```python
from build123d import *

# Parameters (mm, degrees)
F1_DEPTH    = 15
F2_T1_DEPTH = 34.8219363514
F2_T3_DEPTH = 25.2867319519
F2_T5_DEPTH = 87.7867319519
F3_R        = 5
F4_SIZE     = 1


# Not quite as in the source:
# - a fillet or chamfer that OpenCascade refuses, or shapes differently, is made with other operations: its cross-section is extruded or revolved along the edge and cut away or added


with BuildPart() as f1:
    # F0 (on Front) → F1 (new body)
    with BuildSketch(Plane.XZ):
        with BuildLine():
            Line((50, 60), (0, 60))
            Line((0, 60), (-27.5, 60))
            Line((-27.5, 60), (-27.5, 29.0612040202))
            Line((-27.5, 29.0612040202), (-10.1093475479, 5.1480552127))
            ThreePointArc((-10.1093475479, 5.1480552127), (0, 0), (10.1093475479, 5.1480552127))
            Line((10.1093475479, 5.1480552127), (50, 60))
        make_face()
        with BuildLine():
            ThreePointArc((12.5, 32.5), (-8.8388347648, 23.6611652352), (0, 45))
            ThreePointArc((0, 45), (8.8388347648, 41.3388347648), (12.5, 32.5))
        make_face(mode=Mode.SUBTRACT)
    extrude(amount=F1_DEPTH)

    # F2: chamfer of 2 on 7 edges, made by hand

    # F2_s2 → F2_t1 (cut)
    with BuildSketch(Plane.XZ.offset(-9.9109681757)):
        Polygon((47.69005228, 56.823688834), (46.0725566723, 60), (50, 60), align=None)
    extrude(amount=F2_T1_DEPTH, mode=Mode.SUBTRACT)

    # F2_s4 → F2_t3 (cut)
    with BuildSketch(Plane.XZ.offset(-5.1433659759)):
        Polygon((-25.5, 60), (-27.5, 58), (-27.5, 60), align=None)
    extrude(amount=F2_T3_DEPTH, mode=Mode.SUBTRACT)

    # F2_s6 → F2_t5 (cut)
    with BuildSketch(Plane.YZ.offset(-32.6433659759)):
        Polygon((-2, 60), (0, 58), (0, 60), align=None)
        Polygon((-13, 60), (-15, 58), (-15, 60), align=None)
    extrude(amount=F2_T5_DEPTH, mode=Mode.SUBTRACT)

    # F2_s7 → F2_t8 (revolve, cut)
    with BuildSketch(Plane.XY.offset(32.5)):
        Polygon((12.5, -2), (14.5, 0), (12.5, 0), align=None)
    revolve(axis=Axis((0, 0, 32.5), (0, 1, 0)), mode=Mode.SUBTRACT)

    # F2_s9 → F2_t10 (revolve, cut)
    with BuildSketch(Plane.XY.offset(32.5)):
        Polygon((12.5, -13), (14.5, -15), (12.5, -15), align=None)
    revolve(axis=Axis((0, -15, 32.5), (0, 1, 0)), mode=Mode.SUBTRACT)

    # F3
    f3_edges = [f1.edges().sort_by_distance(p)[0] for p in [
        (-27.5, -7.5, 29.061204),
    ]]
    fillet(f3_edges, radius=F3_R)

    # F4
    f4_edges = [f1.edges().sort_by_distance(p)[0] for p in [
        (28.8997, -15, 30.985872),
        (28.8997, 0, 30.985872),
        (-27.5, 0, 44.343534),
        (-27.254929, 0, 29.140895),
        (-18.326543, 0, 16.447173),
        (0, 0, 0),
        (-27.5, -15, 44.343534),
        (-27.254929, -15, 29.140895),
        (-18.326543, -15, 16.447173),
        (0, -15, 0),
    ]]
    chamfer(f4_edges, length=F4_SIZE)


solid = f1.part
```
For this review, take the finished solid that the model builds, in its own axes (mm). Round coordinates to 2 decimals unless told otherwise and drop trailing zeros. Order: outer loops, then holes, each group sorted by start corner. A loop starts at its lowest first (then second) coordinate and runs counter-clockwise, first axis right, second up.
Q1. Mouldability with a two-part tool opening along Z and no side actions: class faces 1 (the flat face through (46.893, -7.395, 58.39)), 2 (the conical face through (-2.737, -1.875, 44.825)), 3 (the cylindrical face through (-27.26, -7.59, 29.16)), 4 (the conical face through (-2.737, -13.125, 44.825)) as pulls with the +Z half, pulls with the -Z half, needs draft (parallel to the pull), parting line crosses it, or undercut.
Findings below:
face 1: pulls with the +Z half
face 2: undercut
face 3: pulls with the -Z half
face 4: undercut
Q2. We need section C-C, the plane x = 31. Give the boundary of the cut face in (y, z).
Findings below:
outline: (-15, 35.57) - (-14, 33.87) - (-1, 33.87) - (0, 35.57) - (0, 58) - (-2, 60) - (-13, 60) - (-15, 58) - close
Q3. Insertion check: P1, Ø20, axis at x = 0, z = 32.5, coming from the +Y side; P2, Ø6, axis at x = 36, y = -9.5, coming from the -Z side. Each pin has a flat end and moves straight along its axis. Give the tip position at first contact, or say it passes through.
Findings below:
P1: passes through
P2: stops at z = 36.62
Q4. We need section B-B, the plane z = 14.5. Give the boundary of the cut face in (x, y).
Findings below:
outline: (-16.91, -14) - (-15.67, -15) - (15.67, -15) - (16.91, -14) - (16.91, -1) - (15.67, 0) - (-15.67, 0) - (-16.91, -1) - close
Q5. Wall thickness on line 1 (X direction, y = -3.5, z = 38); line 2 (Z direction, x = 6.5, y = -13.75); line 3 (X direction, y = -10.25, z = 32.5): over which ranges is each line inside the solid? List them lowest first.
Findings below:
line 1: x = -27.5 to -11.22, 11.22 to 34
line 2: z = 1.82 to 20.95, 44.05 to 59.25
line 3: x = -27.5 to -12.5, 12.5 to 30
Q6. We need section A-A, the plane y = -7.25. Give the boundary of the cut face in (x, z).
Findings below:
outline: (-27.5, 30.69) arc R5 ccw to (-26.54, 27.75) - (-10.11, 5.15) arc R12.5 ccw to (10.11, 5.15) - (47.69, 56.82) - (46.07, 60) - (-25.5, 60) - (-27.5, 58) - close; hole circle Ø25 at (0, 32.5)
